from build123d import *

# Parameters (mm, degrees)
BOSS_EXTRUDE1_DEPTH             = 3
SKETCH5_W                       = 3
SKETCH5_H                       = 10
CUT_EXTRUDE2_DEPTH              = 100.040395799
CIRPATTERN1_COUNT               = 5
CIRPATTERN1_ANGLE               = 80
CIRPATTERN1_THE_OTHER_WAY_COUNT = 5
CIRPATTERN1_THE_OTHER_WAY_ANGLE = 80


with BuildPart() as part:
    # Sketch4 → Boss-Extrude1 (new body)
    with BuildSketch(Plane.XY):
        with BuildLine():
            Line((70, 0), (-70, 0))
            ThreePointArc((-70, 0), (0, -70), (70, 0))
        make_face()
    extrude(amount=BOSS_EXTRUDE1_DEPTH)

    # Sketch5 → Cut-Extrude2 (cut, through all)
    with BuildSketch(Plane.XY):
        with Locations((0, -65)):
            Rectangle(SKETCH5_W, SKETCH5_H)
    cut_extrude2 = extrude(amount=CUT_EXTRUDE2_DEPTH, mode=Mode.SUBTRACT)

    # CirPattern1: Cut-Extrude2 ×5 about axis
    cirpattern1_axis = Axis((0, 0, 0), (0, 0, -1))
    for i in range(1, CIRPATTERN1_COUNT):
        add(cut_extrude2.rotate(cirpattern1_axis, i * CIRPATTERN1_ANGLE / (CIRPATTERN1_COUNT - 1)), mode=Mode.SUBTRACT)

    # CirPattern1 the other way: Cut-Extrude2 ×5 about axis
    cirpattern1_the_other_way_axis = Axis((0, 0, 0), (0, 0, 1))
    for i in range(1, CIRPATTERN1_THE_OTHER_WAY_COUNT):
        add(cut_extrude2.rotate(cirpattern1_the_other_way_axis, i * CIRPATTERN1_THE_OTHER_WAY_ANGLE / (CIRPATTERN1_THE_OTHER_WAY_COUNT - 1)), mode=Mode.SUBTRACT)


solid = part.part
Geometry: final body of the model. Coordinates: model frame, mm. A direction names the side the tool comes from. Give positions to 0.01 mm unless a question says otherwise; leave off trailing zeros. Loops run counter-clockwise (first coordinate to the right, second up) from the corner with the lowest first, then second, coordinate; pieces in that order, holes last. Notation, with made-up numbers: M -1,75 L 56,75 A5 ccw 56,81 Z; hole C 7.25,-25.75 d1. An arc over 180 degrees is marked long. Put each result on its own line as item: value.
1) Cut plane D-D, the plane x = -15. Return the cut outline in (y, z).
Computed values:
outline: M -68.37,0 L 0,0 L 0,3 L -68.37,3 Z
2) Cut plane C-C, the plane x = -34. Return the cut outline in (y, z).
Computed values:
outline: M -61.19,0 L 0,0 L 0,3 L -61.19,3 Z
3) Reachability of faces 4 (the flat face through (64.33, -9.82, 1.48)), 5 (the cylindrical face through (65.73, -24.08, 1.48)), 6 (the flat face through (0, -60, 1)) from +Z, -Z, +X, -X, +Y, -Y: full face, straight path, thin tool, end or side. Return the list, or none.
Computed values:
face 4: +Z, -Z
face 5: +Z, -Z, +X, -Y
face 6: +Z, -Z, -Y
4) First-contact query: P1, Ø0.9, axis at x = -0.5, z = 2, coming from the -Y side; P2, Ø1.5, axis at x = -41.5, z = 1, coming from the -Y side. Flat tips, straight axial feed; report the tip coordinate or a pass-through.
Computed values:
P1: stops at y = -60
P2: stops at y = -56.92
5) Cut plane B-B, the plane y = -51. Return the cut outline in (x, z).
Computed values:
outline: M -47.95,0 L -44.75,0 L -44.75,3 L -47.95,3 Z; M -40.84,0 L 40.84,0 L 40.84,3 L -40.84,3 Z; M 44.75,0 L 47.95,0 L 47.95,3 L 44.75,3 Z
6) Mould query, pull axis Y, two halves, no side actions, for faces 1 (the flat face through (-20.843, -61.651, 1.479)), 2 (the cylindrical face through (34.87, -60.697, 1.479)), 3 (the flat face through (-1, -27, 3)). Classes: released by +Y, released by -Y, zero draft, split by the parting line, or undercut.
Computed values:
face 1: undercut
face 2: released by -Y
face 3: zero draft
7) Material intervals for L1, parallel to X at y = -48, z = 0.8; L2, parallel to X at y = -64, z = 0.9; L3, parallel to X at y = -50.5, z = 1.75, sorted ascending. Write a range as from..to.
Computed values:
L1: x = -50.95..-42.23, -38.32..38.32, 42.23..50.95
L2: x = -28.35..-24.89, -21.7..-1.5, 1.5..21.7, 24.89..28.35
L3: x = -48.47..-44.33, -40.42..40.42, 44.33..48.47
8) Cut plane A-A, the plane x = 42. Return the cut outline in (y, z).
Computed values:
outline: M -56,0 L -52.39,0 L -52.39,3 L -56,3 Z; M -47.72,0 L 0,0 L 0,3 L -47.72,3 Z
